For this review, take the finished solid that the model builds, in its own axes (mm). A direction names the side the tool comes from. Coordinates: 2 decimals unless noted, no trailing zeros. Order: outer loops, then holes, each group sorted by start corner. A loop starts at its lowest first (then second) coordinate and runs counter-clockwise, first axis right, second up. Notation, with made-up numbers: (-7, 12) - (26, 12) arc R24 cw to (26, 30) - close; hole circle Ø1 at (-23.75, 79). An arc over 180 degrees is marked (long way). One line per item, written item: value. Start each with the question number.
(1) Clearance check with a flat-ended pin moving along its axis: pin 1 (1.5 mm diameter, centred on y = -29.5, z = 16.5, fed in from +X). State where the tip first meets the part, or that it passes through.
(2) Consider section C-C on y = -8. Write out the cut boundary in (x, z), then the cut area to 3 significant figures.
(3) Mouldability with a two-part tool opening along Z and no side actions: class faces 3 (the flat face through (0.977, -27, 32)), 4 (the flat face through (51.777, -44, 31)), 5 (the flat face through (0, -3, 63.5)) as released by +Z, released by -Z, zero draft, split by the parting line, or undercut.
(4) To check wall thickness, follow line 1 along X through (y, z) = (-41, 61.5); line 2 along Y through (x, z) = (41.5, 32); line 3 along X through (y, z) = (-12, 48.5). State the ranges of each line that lie inside material, in increasing order.
(5) Consider section A-A on x = 27. Write out the cut boundary in (y, z).
(6) For faces 1 (the cylindrical face through (-24.8, -6, 32.2)), 2 (the flat face through (26, -49.607, 31)), list the 3-axis set-ups (+Z, -Z, +X, -X, +Y, -Y) from which the entire face can be reached by the end or side of a thin tool; tool diameter is ignored.
(7) Consider section D-D on x = -13.5. Write out the cut boundary in (y, z).
```python
from build123d import *

# Parameters (mm, degrees)
F0_W     = 101.6
F0_H     = 76.2
F1_DEPTH = 63.5
F3_DEPTH = 63.501
F5_DEPTH = 50.8


with BuildPart() as f1:
    # F0 (on Top) → F1 (new body)
    with BuildSketch(Plane.XY):
        with Locations((0.976678, -11.506712)):
            Rectangle(F0_W, F0_H)
    extrude(amount=F1_DEPTH)

    # F2 (on face) → F3 (cut, through all)
    with BuildSketch(Plane.XY.offset(63.5)):
        with BuildLine():
            Line((51.776678, -38.273564), (51.776678, 15.26014))
            ThreePointArc((51.776678, 15.26014), (25.009826, -11.506712), (51.776678, -38.273564))
        make_face()
        with BuildLine():
            ThreePointArc((51.776678, -38.273564), (70.7037, -30.433734), (78.54353, -11.506712))
            ThreePointArc((78.54353, -11.506712), (70.7037, 7.420311), (51.776678, 15.26014))
            Line((51.776678, 15.26014), (51.776678, -38.273564))
        make_face()
    extrude(amount=-F3_DEPTH, mode=Mode.SUBTRACT)

    # F4 (on face) → F5 (cut)
    with BuildSketch(Plane(origin=(-49.823322, 0, 0), x_dir=(0, -1, 0), z_dir=(-1, 0, 0))):
        with BuildLine():
            Line((49.606712, 63.5), (19.711442, 63.5))
            ThreePointArc((19.711442, 63.5), (5.997199, 31.75), (19.711442, 0))
            Line((19.711442, 0), (49.606712, 0))
            Line((49.606712, 0), (49.606712, 63.5))
        make_face()
        with BuildLine():
            ThreePointArc((19.711442, 0), (66.899362, -8.284409), (93.216225, 31.75))
            ThreePointArc((93.216225, 31.75), (66.899362, 71.784409), (19.711442, 63.5))
            Line((19.711442, 63.5), (49.606712, 63.5))
            Line((49.606712, 63.5), (49.606712, 0))
            Line((49.606712, 0), (19.711442, 0))
        make_face()
    extrude(amount=-F5_DEPTH, mode=Mode.SUBTRACT)


solid = f1.part
```
Geometry check:
1. pin 1: stops at x = 32.67
2. outline: (-49.82, 0) - (25.24, 0) - (25.24, 63.5) - (-49.82, 63.5) - (-49.82, 44.81) - (0.98, 44.81) - (0.98, 18.69) - (-49.82, 18.69) - close
2. area: 3,440 mm^2
3. face 3: undercut
3. face 4: zero draft
3. face 5: released by +Z
4. line 1: x = 0.98 to 51.78
4. line 2: y = -49.61 to -36.22, 13.21 to 26.59
4. line 3: x = 0.98 to 25.01
5. outline: (-49.61, 0) - (-21.63, 0) - (-21.63, 63.5) - (-49.61, 63.5) - close; (-1.38, 0) - (26.59, 0) - (26.59, 63.5) - (-1.38, 63.5) - close
6. face 1: -X, -Y
6. face 2: +Z, -Z, +X, -X, -Y
7. outline: (-19.71, 0) - (26.59, 0) - (26.59, 63.5) - (-19.71, 63.5) arc R43.61 cw to start
